Part model, mm, in its own coordinate system. Face numbers are marked on the shaded views. A direction names the side the tool comes from. Give positions to 0.01 mm unless a question says otherwise; leave off trailing zeros. Write each loop counter-clockwise with the first axis right and the second up, starting at its lowest first coordinate (ties: lowest second). Pieces come first, ordered by that corner, then holes. Notation, with made-up numbers: (63.25, 10.25) - (116.25, 10.25) arc R17 ccw to (116.25, 43.25) - close; hole circle Ø8 at (0.25, -6.5). An arc over 180 degrees is marked (long way). Answer in a Markdown table with one row per item. Add a question column.
1. Band-saw the part on D-D on x = -14. Write the cut outline in (y, z).
2. Drop flat-ended pins along their axis: pin 1 Ø3 at (x, y) = (-17, 10.5) entering from +Z; pin 2 Ø0.8 at (x, y) = (4.5, -31.5) entering from +Z. Give the stop position or say it passes through.
3. Which spindle directions (+Z, -Z, +X, -X, +Y, -Y) get a long thin tool onto all of the face, cutting with end or side? Do the marked faces 4 and 5. Say none if no direction does.
4. Band-saw the part on C-C on z = 4. Write the cut outline in (x, y).
5. Band-saw the part on B-B on y = -20.5. Write the cut outline in (x, z).
6. Probe line 1 along Y through (x, z) = (19, 11.25); line 2 along X through (y, z) = (14, 24.5); line 3 along Z through (x, y) = (-8, -29). List the from-to ranges inside material, lowest first.
7. Pull direction X, two halves, no side cores. Call the marked faces 1, 2 and 3: released by +X, released by -X, zero draft, split by the parting line, or undercut.
8. Band-saw the part on A-A on z = 11.5. Write the cut outline in (x, y).
```python
from build123d import *

# Parameters (mm, degrees)
F0_W     = 70
F0_H     = 64
F1_DEPTH = 2
F2_W     = 70
F2_H     = 64
F2_W_2   = 68
F2_H_2   = 62
F3_DEPTH = 25
F5_DEPTH = 125


with BuildPart() as f1:
    # F0 (on Top) → F1 (new body)
    with BuildSketch(Plane.XY):
        Rectangle(F0_W, F0_H)
    extrude(amount=F1_DEPTH)

    # F2 (on face) → F3 (join)
    with BuildSketch(Plane.XY.offset(2)):
        Rectangle(F2_W, F2_H)
        Rectangle(F2_W_2, F2_H_2, mode=Mode.SUBTRACT)
    extrude(amount=F3_DEPTH)

    # F4 (on face) → F5 (cut)
    with BuildSketch(Plane.XZ.offset(32)):
        with BuildLine():
            Line((-10, 7), (0, 7))
            Line((0, 7), (10, 7))
            Line((10, 7), (10, 17))
            ThreePointArc((10, 17), (12.928932, 24.071068), (20, 27))
            Line((20, 27), (-20, 27))
            ThreePointArc((-20, 27), (-12.928932, 24.071068), (-10, 17))
            Line((-10, 17), (-10, 7))
        make_face()
    extrude(amount=-F5_DEPTH, mode=Mode.SUBTRACT)


solid = f1.part
```
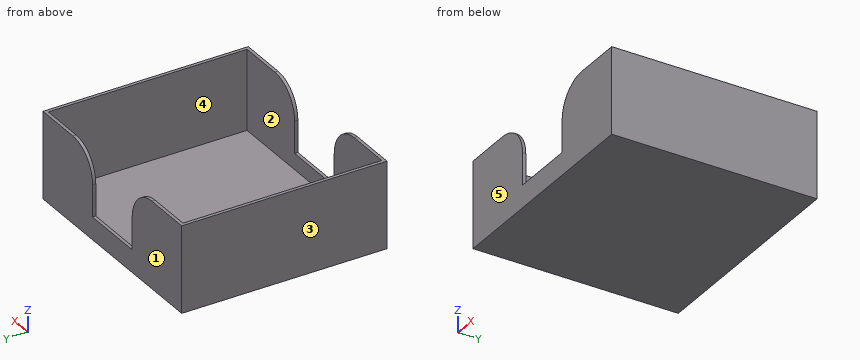
Values:
| question | item | result |
|---|---|---|
| 1 | outline | (-32, 0) - (32, 0) - (32, 25) - (31, 25) - (31, 2) - (-31, 2) - (-31, 25) - (-32, 25) - close |
| 2 | pin 1 | stops at z = 2 |
| 2 | pin 2 | stops at z = 7 |
| 3 | face 4 | +Z |
| 3 | face 5 | +Z, -Z, +X, -X, -Y |
| 4 | outline | (-35, -32) - (35, -32) - (35, 32) - (-35, 32) - close; hole (-34, -31) - (34, -31) - (34, 31) - (-34, 31) - close |
| 5 | outline | (-35, 0) - (35, 0) - (35, 27) - (34, 27) - (34, 2) - (-34, 2) - (-34, 27) - (-35, 27) - close |
| 6 | line 1 | y = -32 to -31, 31 to 32 |
| 6 | line 2 | x = -35 to -34, 34 to 35 |
| 6 | line 3 | z = 0 to 2 |
| 7 | face 1 | zero draft |
| 7 | face 2 | undercut |
| 7 | face 3 | released by -X |
| 8 | outline | (-35, -32) - (-10, -32) - (-10, -31) - (-34, -31) - (-34, 31) - (-10, 31) - (-10, 32) - (-35, 32) - close; (10, -32) - (35, -32) - (35, 32) - (10, 32) - (10, 31) - (34, 31) - (34, -31) - (10, -31) - close |
